from build123d import *

# Parameters (mm, degrees)
ESBO_O1_W                = 115
ESBO_O1_H                = 225
RESSALTO_EXTRUS_O1_DEPTH = 15
ESBO_O2_R                = 5
CORTE_EXTRUS_O1_DEPTH    = 254.130401177


with BuildPart() as part:
    # Esboço1 → Ressalto-extrusão1 (new body)
    with BuildSketch(Plane.XY):
        with Locations((57.5, 112.5)):
            Rectangle(ESBO_O1_W, ESBO_O1_H)
    extrude(amount=RESSALTO_EXTRUS_O1_DEPTH)

    # Esboço2 → Corte-extrusão1 (cut, through all)
    with BuildSketch(Plane.XY.offset(15)):
        with Locations((57.5, 190)):
            Circle(ESBO_O2_R)
        with Locations((57.5, 112.5)):
            Circle(ESBO_O2_R)
        with Locations(Location((57.5, 35, 0), (0, 0, 180))):
            Circle(ESBO_O2_R)
    extrude(amount=-CORTE_EXTRUS_O1_DEPTH, mode=Mode.SUBTRACT)


solid = part.part
Build history of the part. All positions in model axes, mm. Round coordinates to 2 decimals unless told otherwise and drop trailing zeros. Write each loop counter-clockwise with the first axis right and the second up, starting at its lowest first coordinate (ties: lowest second). Pieces come first, ordered by that corner, then holes. Notation, with made-up numbers: M 61,45.5 L 98,45.5 A8 cw 98,58.5 Z; hole C -27,-40 d5. An arc over 180 degrees is marked long. Answer as a JSON object with one key per item and string values. Group by question number.
(1) Flat gauge pin, fed straight in: pin 1 (8 mm diameter, centred on x = 57.5, y = 112.5, fed in from -Z). Where does the tip first touch, or does it go through?
(2) Cut at B-B (x = 57.5). Give the cut face in (y, z), and give its area (4 significant figures).
(3) Cut at A-A (y = 112.5). Give the cut face in (x, z).
(4) Drill centre lines: L1, parallel to Y at x = 57.5, z = 8.75; L2, parallel to X at y = 35, z = 8.75. Where is each one in solid material? Low to high.
(5) Mould opens along Y. For faces 1 (the flat face through (57, 225, 7)), 2 (the cylindrical face through (56.849, 194.957, 7.605)), 3 (the flat face through (0, 111, 7)) say: pulls with the +Y half, pulls with the -Y half, needs draft (parallel to the pull), parting line crosses it, or undercut.
Responses:
{
 "1": {"pin 1": "passes through"},
 "2": {"outline": "M 0,0 L 30,0 L 30,15 L 0,15 Z; M 40,0 L 107.5,0 L 107.5,15 L 40,15 Z; M 117.5,0 L 185,0 L 185,15 L 117.5,15 Z; M 195,0 L 225,0 L 225,15 L 195,15 Z", "area": "2,925 mm2"},
 "3": {"outline": "M 0,0 L 52.5,0 L 52.5,15 L 0,15 Z; M 62.5,0 L 115,0 L 115,15 L 62.5,15 Z"},
 "4": {"L1": "y = 0 to 30, 40 to 107.5, 117.5 to 185, 195 to 225", "L2": "x = 0 to 52.5, 62.5 to 115"},
 "5": {"face 1": "pulls with the +Y half", "face 2": "undercut", "face 3": "needs draft"}
}
